Could you check a few things on this model? Use its own coordinates, in mm. A direction names the side the tool comes from. Give positions to 0.01 mm unless a question says otherwise; leave off trailing zeros. Order: outer loops, then holes, each group sorted by start corner. A loop starts at its lowest first (then second) coordinate and runs counter-clockwise, first axis right, second up. Notation, with made-up numbers: M 36.25,-24 L 60.25,-24 A7 cw 60.25,-17 Z; hole C 21.5,31 d2. An arc over 180 degrees is marked long. Use a Markdown table: item, result. Add a question column.
Item 1: If I drill on L1, parallel to Y at x = 0, z = 0.65; L2, parallel to Y at x = -5, z = 1.55; L3, parallel to Y at x = -31, z = 1.25, over which ranges is the centre line in solid material (lowest first)? Write a range as from..to.
Item 2: For faces 5 (the face through (38.678, 0, 1)), 6 (the face through (24.16, 17.95, -2.28)), which set-ups out of +Z, -Z, +X, -X, +Y, -Y let a thin tool reach every point of the face, with its end or its side?
Item 3: I'm going to push flat-ended pins straight in: pin 1 Ø3 at (y, z) = (-23.5, -4) entering from -X; pin 2 Ø3.5 at (x, y) = (5, 30.678) entering from -Z; pin 3 Ø1.5 at (x, z) = (-25, 0) entering from -Y. Where does each tip first touch, or does it pass through?
Item 4: If we mould it in two halves opening along Y, with no side actions, what happens to faces 1 (the face through (0, -38.678, 1)), 2 (the face through (18.301, -26.603, 0.986)), 3 (the face through (-17.95, -24.16, -2.28)), 4 (the face through (18, -23, -6.679))? For each: released by +Y, released by -Y, zero draft, split by the parting line, or undercut.
Item 5: Suppose I cut it at C-C on z = -2.5. Write out the boundary of the cut face in (x, y), plus the area to 3 significant figures.
Item 6: Suppose I cut it at A-A on x = -5. Write out the boundary of the cut face in (y, z).
Item 7: Suppose I cut it at B-B on y = 0. Write out the boundary of the cut face in (x, z), plus the area to 3 significant figures.
Autodesk Inventor part; units mm, degrees
ref_plane "РабПлоскость1" through (-27.178, -27.178, -6.6792) normal (0, 0, 1) x (1, 0, 0)
ref_plane "YZ Plane" through (0, 0, 0) normal (1, 0, 0) x (0, 1, 0)
ref_plane "XZ Plane" through (0, 0, 0) normal (0, 1, 0) x (-1, 0, 0)
sketch "Эскиз1" plane through (0, 0, 0) normal (0, 0, 1) x (1, 0, 0)
  line L0 (-28.678, -17.6393) -> (-17.6393, -28.678) construction
  line L1 (-17.6393, -28.678) -> (-7, -28.678) construction
  line L2 (-7, -32.678) -> (-7, -28.678) construction
  line L3 (-3, -32.678) -> (-7, -32.678) construction
  line L4 (-3, -28.678) -> (-3, -32.678) construction
  line L5 (-3, -28.678) -> (17.6393, -28.678) construction
  line L6 (17.6393, -28.678) -> (28.678, -17.6393) construction
  line L7 (28.678, -17.6393) -> (28.678, -7) construction
  line L8 (32.678, -7) -> (28.678, -7) construction
  line L9 (32.678, -3) -> (32.678, -7) construction
  line L10 (28.678, -3) -> (32.678, -3) construction
  line L11 (28.678, -3) -> (28.678, 17.6393) construction
  line L12 (28.678, 17.6393) -> (17.6393, 28.678) construction
  line L13 (17.6393, 28.678) -> (7, 28.678) construction
  line L14 (7, 32.678) -> (7, 28.678) construction
  line L15 (3, 32.678) -> (7, 32.678) construction
  line L16 (3, 28.678) -> (3, 32.678) construction
  line L17 (3, 28.678) -> (-17.6393, 28.678) construction
  line L18 (-17.6393, 28.678) -> (-28.678, 17.6393) construction
  line L19 (-28.678, 17.6393) -> (-28.678, 7) construction
  line L20 (-32.678, 7) -> (-28.678, 7) construction
  line L21 (-32.678, 3) -> (-32.678, 7) construction
  line L22 (-28.678, 3) -> (-32.678, 3) construction
  line L23 (-28.678, 3) -> (-28.678, -17.6393) construction
  line L24 (-27.678, 17.2251) -> (-17.2251, 27.678) construction
  line L25 (-17.2251, 27.678) -> (17.2251, 27.678) construction
  line L26 (17.2251, 27.678) -> (27.678, 17.2251) construction
  line L27 (27.678, 17.2251) -> (27.678, -17.2251) construction
  line L28 (27.678, -17.2251) -> (17.2251, -27.678) construction
  line L29 (17.2251, -27.678) -> (-17.2251, -27.678) construction
  line L30 (-17.2251, -27.678) -> (-27.678, -17.2251) construction
  line L31 (-27.678, -17.2251) -> (-27.678, 17.2251) construction
  line L32 (38.678, 21.7815) -> (21.7815, 38.678)
  line L33 (21.7815, 38.678) -> (-21.7815, 38.678)
  line L34 (-21.7815, 38.678) -> (-38.678, 21.7815)
  line L35 (-38.678, 21.7815) -> (-38.678, -21.7815)
  line L36 (-38.678, -21.7815) -> (-21.7815, -38.678)
  line L37 (-21.7815, -38.678) -> (21.7815, -38.678)
  line L38 (21.7815, -38.678) -> (38.678, -21.7815)
  line L39 (38.678, -21.7815) -> (38.678, 21.7815)
  line L40 (17.2251, 27.678) -> (27.678, 17.2251)
  line L41 (27.678, 17.2251) -> (27.678, -17.2251)
  line L42 (27.678, -17.2251) -> (17.2251, -27.678)
  line L43 (17.2251, -27.678) -> (-17.2251, -27.678)
  line L44 (-17.2251, -27.678) -> (-27.678, -17.2251)
  line L45 (-27.678, -17.2251) -> (-27.678, 17.2251)
  line L46 (-27.678, 17.2251) -> (-17.2251, 27.678)
  line L47 (-17.2251, 27.678) -> (17.2251, 27.678)
  circle A0 centre (30.678, -5) radius 1.5
  circle A1 centre (5, 30.678) radius 1.5
  circle A2 centre (-30.678, 5) radius 1.5
  circle A3 centre (-5, -30.678) radius 1.5
  circle A4 centre (5, 30.678) radius 1
  circle A5 centre (-30.678, 5) radius 1
  circle A6 centre (30.678, -5) radius 1
  circle A7 centre (-5, -30.678) radius 1
  point P0 (0, 0)
  dimension "d0" = 11
  dimension "d1" = 11
  dimension "d4" = 3
  dimension "d5" = 3
  dimension "d6" = 3
  dimension "d7" = 3
extrude "Выдавливание2" add sketch "Эскиз1" along normal blind 2 contours L39 L38 L37 L36 L35 L34 L33 L32
sketch "Эскиз2" plane through (0, 0, 2) normal (0, 0, 1) x (1, 0, 0)
  line L0 (21.7815, 38.678) -> (-21.7815, 38.678) construction
  line L1 (-21.7815, 38.678) -> (-38.678, 21.7815) construction
  line L2 (-38.678, 21.7815) -> (-38.678, -21.7815) construction
  line L3 (-38.678, -21.7815) -> (-21.7815, -38.678) construction
  line L4 (-21.7815, -38.678) -> (21.7815, -38.678) construction
  line L5 (21.7815, -38.678) -> (38.678, -21.7815) construction
  line L6 (38.678, -21.7815) -> (38.678, 21.7815) construction
  line L7 (38.678, 21.7815) -> (21.7815, 38.678) construction
  line L8 (17.2251, 27.678) -> (27.678, 17.2251) construction
  line L9 (27.678, 17.2251) -> (27.678, -17.2251) construction
  line L10 (27.678, -17.2251) -> (17.2251, -27.678) construction
  line L11 (17.2251, -27.678) -> (-17.2251, -27.678) construction
  line L12 (-17.2251, -27.678) -> (-27.678, -17.2251) construction
  line L13 (-27.678, -17.2251) -> (-27.678, 17.2251) construction
  line L14 (-27.678, 17.2251) -> (-17.2251, 27.678) construction
  line L15 (-17.2251, 27.678) -> (17.2251, 27.678) construction
  circle A0 centre (-5, -30.678) radius 1.5 construction
  circle A1 centre (-30.678, 5) radius 1.5 construction
  circle A2 centre (5, 30.678) radius 1.5 construction
  circle A3 centre (30.678, -5) radius 1.5 construction
  line L16 (27.678, -17.2251) -> (17.2251, -27.678)
  line L17 (22.1749, -22.7283) -> (19.3464, -25.5567)
  line L18 (19.3464, -25.5567) -> (16.518, -22.7283)
  line L19 (16.518, -22.7283) -> (19.3464, -19.8998)
  line L20 (19.3464, -19.8998) -> (22.1749, -22.7283)
  line L21 (17.2251, -27.678) -> (-17.2251, -27.678) construction
  line L22 (0, -27.678) -> (0, 27.678) construction
  line L23 (27.678, 17.2251) -> (27.678, -17.2251) construction
  line L24 (27.678, 0) -> (-27.678, 0) construction
  line L25 (-27.678, -17.2251) -> (-27.678, 17.2251) construction
  line L26 (-22.1749, -22.7283) -> (-19.3464, -25.5567)
  line L27 (-19.3464, -25.5567) -> (-16.518, -22.7283)
  line L28 (-16.518, -22.7283) -> (-19.3464, -19.8998)
  line L29 (-19.3464, -19.8998) -> (-22.1749, -22.7283)
  line L30 (-27.678, 17.2251) -> (-17.2251, 27.678) construction
  line L31 (22.4516, -22.4516) -> (-22.4516, 22.4516) construction
  line L32 (27.678, 17.2251) -> (17.2251, 27.678) construction
  line L33 (22.7283, 22.1749) -> (25.5567, 19.3464)
  line L34 (19.8998, 19.3464) -> (22.7283, 22.1749)
  line L35 (22.7283, 16.518) -> (19.8998, 19.3464)
  line L36 (25.5567, 19.3464) -> (22.7283, 16.518)
  circle A4 centre (19.3407, -22.734) radius 1
  circle A5 centre (-19.3738, -22.7283) radius 1
  circle A6 centre (22.7283, 19.3419) radius 1
  line L37 (-23.1587, 16.0876) -> (-20.3302, 18.916)
  line L38 (-20.3302, 18.916) -> (-23.1587, 21.7444)
  line L39 (-23.1587, 21.7444) -> (-25.9871, 18.916)
  line L40 (-25.9871, 18.916) -> (-23.1587, 16.0876)
  circle A7 centre (-23.1587, 18.9654) radius 1
  point P0 (0, 0)
  dimension "d11" = 4
  dimension "d12" = 3
  dimension "d30" = 2
  dimension "d31" = 2
  dimension "d32" = 2
  dimension "d33" = 4
  dimension "d34" = 4
  dimension "d36" = 1
  dimension "d37" = 2
ref_plane "РабПлоскость1" through (-27.178, -27.178, -6.6792) normal (0, 0, 1) x (1, 0, 0)
extrude "Выдавливание3" add sketch "Эскиз2" against normal up to surface (8.6792 mm away)
sketch "Эскиз3" plane through (0, 0, 2) normal (0, 0, 1) x (1, 0, 0)
  circle A0 centre (-5, -30.678) radius 1.5 construction
  circle A1 centre (30.678, -5) radius 1.5 construction
  circle A2 centre (-30.678, 5) radius 1.5 construction
  circle A3 centre (5, 30.678) radius 1.5 construction
  line L0 (-17.2251, 27.678) -> (17.2251, 27.678) construction
  line L1 (0, 27.678) -> (0, -27.678) construction
  line L2 (17.2251, -27.678) -> (-17.2251, -27.678) construction
  line L3 (27.678, 17.2251) -> (27.678, -17.2251) construction
  line L4 (27.678, 0) -> (-27.678, 0) construction
  line L5 (-27.678, -17.2251) -> (-27.678, 17.2251) construction
  circle A4 centre (0, -31.678) radius 1.5
  circle A5 centre (31.678, 0) radius 1.5
  circle A6 centre (-31.678, 0) radius 1.5
  circle A7 centre (0, 31.678) radius 1.5
  point P0 (0, 0)
  dimension "d15" = 3
  dimension "d16" = 3
  dimension "d17" = 3
  dimension "d18" = 3
  dimension "d19" = 4
  dimension "d20" = 4
  dimension "d21" = 4
  dimension "d22" = 4
extrude "Выдавливание4" cut sketch "Эскиз3" against normal through all
properties part number "Середина"
Findings below:
| question | item | result |
|---|---|---|
| 1 | L1 | y = -38.68..-33.18, -30.18..-27.68, 27.68..30.18, 33.18..38.68 |
| 1 | L2 | y = -38.68..-32.18, -29.18..-27.68, 27.68..38.68 |
| 1 | L3 | y = -29.46..-1.34, 1.34..3.53, 6.47..29.46 |
| 2 | face 5 | +Z, -Z, +X, +Y, -Y |
| 2 | face 6 | +Z, -Z |
| 3 | pin 1 | stops at x = -22.17 |
| 3 | pin 2 | stops at z = 0 |
| 3 | pin 3 | stops at y = -36.21 |
| 4 | face 1 | released by -Y |
| 4 | face 2 | undercut |
| 4 | face 3 | undercut |
| 4 | face 4 | zero draft |
| 5 | outline | M -25.99,18.92 L -23.16,16.09 L -20.33,18.92 L -23.16,21.74 Z; M -22.17,-22.73 L -19.35,-25.56 L -16.52,-22.73 L -19.35,-19.9 Z; M 16.52,-22.73 L 19.35,-25.56 L 22.17,-22.73 L 19.35,-19.9 Z; M 19.9,19.35 L 22.73,16.52 L 25.56,19.35 L 22.73,22.17 Z; hole C -23.16,18.97 d2; hole C -19.37,-22.73 d2; hole C 19.34,-22.73 d2; hole C 22.73,19.34 d2 |
| 5 | area | 51.4 mm^2 |
| 6 | outline | M -38.68,0 L -32.18,0 L -32.18,2 L -38.68,2 Z; M -29.18,0 L -27.68,0 L -27.68,2 L -29.18,2 Z; M 27.68,0 L 38.68,0 L 38.68,2 L 27.68,2 Z |
| 7 | outline | M -38.68,0 L -33.18,0 L -33.18,2 L -38.68,2 Z; M -30.18,0 L -27.68,0 L -27.68,2 L -30.18,2 Z; M 27.68,0 L 30.18,0 L 30.18,2 L 27.68,2 Z; M 33.18,0 L 38.68,0 L 38.68,2 L 33.18,2 Z |
| 7 | area | 32.0 mm^2 |
